```python
from build123d import *

# Parameters (mm, degrees)
F0_R     = 35
F1_DEPTH = 6
F2_R     = 1.55
F3_DEPTH = 6.001
F4_R     = 25
F5_DEPTH = 6.001


with BuildPart() as f1:
    # F0 (on Top) → F1 (new body)
    with BuildSketch(Plane.XY):
        Circle(F0_R)
    extrude(amount=F1_DEPTH)

    # F2 (on face) → F3 (cut, through all)
    with BuildSketch(Plane.XY.offset(6)):
        with Locations((0, 30)):
            Circle(F2_R)
        with Locations((-25.980762, 15)):
            Circle(F2_R)
        with Locations((-25.980762, -15)):
            Circle(F2_R)
        with Locations((25.980762, 15)):
            Circle(F2_R)
        with Locations((25.980762, -15)):
            Circle(F2_R)
        with Locations((0, -30)):
            Circle(F2_R)
    extrude(amount=-F3_DEPTH, mode=Mode.SUBTRACT)

    # F4 (on face) → F5 (cut, through all)
    with BuildSketch(Plane.XY.offset(6)):
        Circle(F4_R)
    extrude(amount=-F5_DEPTH, mode=Mode.SUBTRACT)


solid = f1.part
```
CAD build for the part. Positions are in the model's coordinates, mm. Round coordinates to 2 decimals unless told otherwise and drop trailing zeros. Order: outer loops, then holes, each group sorted by start corner. A loop starts at its lowest first (then second) coordinate and runs counter-clockwise, first axis right, second up. Notation, with made-up numbers: (-8.75, 29.25) -> (30.25, 29.25) arc R26 cw to (30.25, 58.25) -> close; hole circle Ø8 at (22, 30). An arc over 180 degrees is marked (long way). Write item = value, one per line.
(1) Drill centre lines: L1, parallel to Y at x = 0, z = 4.5; L2, parallel to Y at x = -1, z = 0.8; L3, parallel to Y at x = -25.5, z = 1.65. Where is each one in solid material? Low to high.
Answers follow:
L1 = -35 to -31.55, -28.45 to -25, 25 to 28.45, 31.55 to 35
L2 = -34.99 to -31.18, -28.82 to -24.98, 24.98 to 28.82, 31.18 to 34.99
L3 = -23.97 to -16.47, -13.53 to 13.53, 16.47 to 23.97
(2) Cut at A-A (x = 0). Write the cut outline in (y, z).
Answers follow:
outline = (-35, 0) -> (-31.55, 0) -> (-31.55, 6) -> (-35, 6) -> close; (-28.45, 0) -> (-25, 0) -> (-25, 6) -> (-28.45, 6) -> close; (25, 0) -> (28.45, 0) -> (28.45, 6) -> (25, 6) -> close; (31.55, 0) -> (35, 0) -> (35, 6) -> (31.55, 6) -> close
(3) Cut at B-B (y = 0). Write the cut outline in (x, z), plus the area to 3 significant figures.
Answers follow:
outline = (-35, 0) -> (-25, 0) -> (-25, 6) -> (-35, 6) -> close; (25, 0) -> (35, 0) -> (35, 6) -> (25, 6) -> close
area = 120 mm²
(4) Cut at C-C (z = 4.3). Write the cut outline in (x, y), plus the area to 3 significant figures.
Answers follow:
outline = circle Ø70 at (0, 0); hole circle Ø3.1 at (-25.98, -15); hole circle Ø3.1 at (-25.98, 15); hole circle Ø50 at (0, 0); hole circle Ø3.1 at (0, -30); hole circle Ø3.1 at (0, 30); hole circle Ø3.1 at (25.98, -15); hole circle Ø3.1 at (25.98, 15)
area = 1,840 mm²
(5) Pull direction X, two halves, no side cores. Call faces 1 (the cylindrical face through (-28, -21, 3)), 2 (the cylindrical face through (26.81, -13.69, 3.04)), 3 (the cylindrical face through (26.81, 16.31, 3.04)), 4 (the flat face through (23.2, -10.2, 0)): +X half, -X half, draft (parallel to the pull), parting line (faces both ways), or undercut.
Answers follow:
face_1 = parting line
face_2 = undercut
face_3 = undercut
face_4 = draft
(6) Cut at D-D (x = 9). Write the cut outline in (y, z).
Answers follow:
outline = (-33.82, 0) -> (-23.32, 0) -> (-23.32, 6) -> (-33.82, 6) -> close; (23.32, 0) -> (33.82, 0) -> (33.82, 6) -> (23.32, 6) -> close
(7) Flat gauge pins, fed straight in: P1, Ø2, axis at y = 19.5, z = 3, coming from the -X side; P2, Ø3.5, axis at x = 0, y = -30, coming from the -Z side. Where does each tip first touch, or does it go through?
Answers follow:
P1 = -29.71
P2 = 0
